from build123d import *

# Parameters (mm, degrees)
SKETCH1_W           = 15.24
SKETCH1_H           = 10.16
BOSS_EXTRUDE1_DEPTH = 4
BOSS_EXTRUDE2_DEPTH = 10.16
SKETCH3_R           = 3.81
CUT_EXTRUDE1_DEPTH  = 3


with BuildPart() as part:
    # Sketch1 → Boss-Extrude1 (new body)
    with BuildSketch(Plane(origin=(0, 0, 0), x_dir=(1, 0, 0), z_dir=(0, 1, 0))):
        Rectangle(SKETCH1_W, SKETCH1_H)
    extrude(amount=BOSS_EXTRUDE1_DEPTH)

    # Sketch2 → Boss-Extrude2 (add)
    with BuildSketch(Plane.XY.offset(5.08)):
        with BuildLine():
            Line((13.62, 4), (7.62, 4))
            Line((7.62, 4), (7.62, 0))
            Line((7.62, 0), (13.62, 0))
            ThreePointArc((13.62, 0), (23.535142279, -1.740916975), (33.025, -5.1))
            Line((33.025, -5.1), (39.965, -5.1))
            ThreePointArc((39.965, -5.1), (27.323058228, 0.985995221), (13.62, 4))
        make_face()
        with BuildLine():
            Line((-7.62, 0), (-7.62, 4))
            Line((-7.62, 4), (-13.62, 4))
            ThreePointArc((-13.62, 4), (-27.323058228, 0.985995221), (-39.965, -5.1))
            Line((-39.965, -5.1), (-33.025, -5.1))
            ThreePointArc((-33.025, -5.1), (-23.535142279, -1.740916975), (-13.62, 0))
            Line((-13.62, 0), (-7.62, 0))
        make_face()
    extrude(amount=-BOSS_EXTRUDE2_DEPTH)

    # Sketch3 → Cut-Extrude1 (cut)
    with BuildSketch(Plane(origin=(0, 4, 0), x_dir=(1, 0, 0), z_dir=(0, 1, 0))):
        Circle(SKETCH3_R)
    extrude(amount=-CUT_EXTRUDE1_DEPTH, mode=Mode.SUBTRACT)


solid = part.part
The model under review builds one solid part; all positions refer to its coordinate system, in mm. A direction names the side the tool comes from. Give positions to 0.01 mm unless a question says otherwise; leave off trailing zeros. Loops run counter-clockwise (first coordinate to the right, second up) from the corner with the lowest first, then second, coordinate; pieces in that order, holes last. Notation, with made-up numbers: (30, 84) -> (65, 84) arc R13 cw to (65, 95) -> close; hole circle Ø3 at (53.25, 88). An arc over 180 degrees is marked (long way). Answer as a JSON object with one key per item and string values. Group by question number.
Q1. Take a section at A-A (z = 0). Write out the cut boundary in (x, y) (1 decimal), plus the area to 3 significant figures.
Q2. Draft analysis for pull direction X (two halves, no side actions). For faces 4 (the flat face through (36, -5.1, 0)), 5 (the cylindrical face through (27.51, 0.92, 0.07)), 6 (the flat face through (0, 1, 0)), state which applies: pulls with the +X half, pulls with the -X half, needs draft (parallel to the pull), parting line crosses it, or undercut.
Q3. Insertion check: pin 1 (1 mm diameter, centred on x = -17, z = 1, fed in from -Y); pin 2 (1.5 mm diameter, centred on y = -2.5, z = -2.5, fed in from -X); pin 3 (6 mm diameter, centred on x = 5.5, z = 3, fed in from -Y). Each pin has a flat end and moves straight along its axis. Give the tip position at first contact, or say it passes through.
Q4. Take a section at B-B (x = 0). Write out the cut boundary in (y, z).
Q5. Take a section at D-D (y = 2.75). Write out the cut boundary in (x, z).
Q6. Wall thickness on line 1 along Z through (x, y) = (0, 2.3); line 2 along Y through (x, z) = (-3, -3.5); line 3 along Y through (x, z) = (-1.5, -1.25): over which ranges is each line inside the solid? List them lowest first.
Q7. Take a section at C-C (y = -2). Write out the cut boundary in (x, z).
Q8. Tool access review of faces 1 (the flat face through (-1, 1, 5.08)), 2 (the cylindrical face through (-0.83, 2.52, 3.72)), 3 (the cylindrical face through (-23.672, -1.777, 0.071)): name each direction out of +Z, -Z, +X, -X, +Y, -Y from which nothing blocks a thin tool from reaching the whole face with its end or side.
Answer below:
{
 "1": {"outline": "(-40, -5.1) -> (-33, -5.1) arc R60.6 cw to (-13.6, 0) -> (13.6, 0) arc R60.6 cw to (33, -5.1) -> (40, -5.1) arc R60.6 ccw to (13.6, 4) -> (3.8, 4) -> (3.8, 1) -> (-3.8, 1) -> (-3.8, 4) -> (-13.6, 4) arc R60.6 ccw to start", "area": "265 mm2"},
 "2": {"face 4": "needs draft", "face 5": "pulls with the +X half", "face 6": "undercut"},
 "3": {"pin 1": "stops at y = -0.48", "pin 2": "stops at x = -36.84", "pin 3": "stops at y = 0"},
 "4": {"outline": "(0, -5.08) -> (4, -5.08) -> (4, -3.81) -> (1, -3.81) -> (1, 3.81) -> (4, 3.81) -> (4, 5.08) -> (0, 5.08) -> close"},
 "5": {"outline": "(-21.18, -5.08) -> (21.18, -5.08) -> (21.18, 5.08) -> (-21.18, 5.08) -> close; hole circle Ø7.62 at (0, 0)"},
 "6": {"line 1": "z = -5.08 to -3.81, 3.81 to 5.08", "line 2": "y = 0 to 4", "line 3": "y = 0 to 1"},
 "7": {"outline": "(-34.46, -5.08) -> (-24.49, -5.08) -> (-24.49, 5.08) -> (-34.46, 5.08) -> close; (24.49, -5.08) -> (34.46, -5.08) -> (34.46, 5.08) -> (24.49, 5.08) -> close"},
 "8": {"face 1": "+Z, +X, -X, +Y, -Y", "face 2": "+Y", "face 3": "+Z, -Z, -Y"}
}
